Check sheet for the modelled part. Datum: model origin and axes. Units: mm. A direction names the side the tool comes from. Coordinates: 2 decimals unless noted, no trailing zeros. Write each loop counter-clockwise with the first axis right and the second up, starting at its lowest first coordinate (ties: lowest second). Pieces come first, ordered by that corner, then holes. Notation, with made-up numbers: (16.5, -11.75) -> (24.5, -11.75) arc R27 cw to (24.5, 9.25) -> close; hole circle Ø7 at (58, 23.25). An arc over 180 degrees is marked (long way). One line per item, written item: value. Start each with the question number.
1) Sectioned sample at B-B on z = 18. Enter the section's corners in (x, y).
2) Set-up check for faces 1 (the flat face through (7.9, -14.4, 0)), 2 (the flat face through (29, 19, 31.5)), 3 (the cylindrical face through (7.262, -32.703, 18.527)): record each of +Z, -Z, +X, -X, +Y, -Y from which the full face is reachable in a straight line by a thin tool's end or side.
3) Gauge pin test, flat ends, axial feed: P1, Ø1, axis at x = 7, z = 11, coming from the +Y side; P2, Ø2, axis at x = -15, z = 8.5, coming from the +Y side; P3, Ø12, axis at y = 8.5, z = 29, coming from the -X side. Record the tip position at first contact, or that the pin passes through.
4) Scan lines: line 1 along Y through (x, z) = (0, 8); line 2 along X through (y, z) = (-4, 14); line 3 along X through (y, z) = (-12.5, 7). Record each from-to range of solid material in increasing order. Write a range as [from, to].
5) Sectioned sample at A-A on z = 6.5. Enter the section's corners in (x, y).
6) Draft check along Z on faces 4 (the conical face through (12.692, -9.732, 3.088)), 5 (the cylindrical face through (-32.907, 10.363, 16.036)), 6 (the flat face through (14, -14, 1)). Enter one of: +Z half, -Z half, draft (parallel to the pull), parting line (faces both ways), or undercut.
```python
from build123d import *

# Parameters (mm, degrees)
F2_R = 1


with BuildPart() as f1:
    # F0 (on Front) → F1 (revolve)
    with BuildSketch(Plane.XZ):
        with BuildLine():
            Line((-33.5, 0), (-16, 0))
            ThreePointArc((-16, 0), (-15.292893, 0.292893), (-15, 1))
            Line((-15, 1), (-15, 17))
            ThreePointArc((-15, 17), (-15.5, 17.013149), (-16, 17))
            Line((-16, 17), (-16, 4.255122))
            Line((-16, 4.255122), (-15.988545, 1.953905))
            ThreePointArc((-15.988545, 1.953905), (-16.142937, 1.325431), (-16.702322, 1))
            ThreePointArc((-16.702322, 1), (-16.805884, 0.993498), (-16.909445, 1))
            Line((-16.909445, 1), (-33.028781, 1))
            ThreePointArc((-33.028781, 1), (-33.360033, 1.216641), (-33.5, 1.586872))
            Line((-33.5, 1.586872), (-33.5, 36))
            Line((-33.5, 36), (-35.5, 36))
            Line((-35.5, 36), (-35.5, 31.5))
            Line((-35.5, 31.5), (-34.5, 31.5))
            Line((-34.5, 31.5), (-34.5, 1))
            ThreePointArc((-34.5, 1), (-34.207107, 0.292893), (-33.5, 0))
        make_face()
    revolve(axis=Axis((0, 0, 10.195818), (0, 0, -1)))

    # F2
    f2_edges = [f1.edges().sort_by_distance(p)[0] for p in [
        (33.5, 0, 36),
    ]]
    fillet(f2_edges, radius=F2_R)


solid = f1.part
```
Answers:
1. outline: circle Ø69 at (0, 0); hole circle Ø67 at (0, 0)
2. face 1: -Z, +X, -X, +Y, -Y
2. face 2: -Z
2. face 3: +Z
3. P1: stops at y = 33.88
3. P2: stops at y = 31.53
3. P3: stops at x = -35.37
4. line 1: y = [-34.5, -33.5], [-16, -15], [15, 16], [33.5, 34.5]
4. line 2: x = [-34.27, -33.26], [-15.49, -14.46], [14.46, 15.49], [33.26, 34.27]
4. line 3: x = [-32.16, -31.08], [-9.99, -8.29], [8.29, 9.99], [31.08, 32.16]
5. outline: circle Ø69 at (0, 0); circle Ø32 at (0, 0); hole circle Ø67 at (0, 0); hole circle Ø30 at (0, 0)
6. face 4: undercut
6. face 5: draft
6. face 6: +Z half
